from build123d import *

# Parameters (mm, degrees)
SKETCH1_W           = 10
SKETCH1_H           = 74.74
SKETCH1_R           = 2.05
BOSS_EXTRUDE1_DEPTH = 85
SKETCH1_2_R         = 2.05
BOSS_EXTRUDE2_DEPTH = 75
SKETCH2_R           = 1.75
CUT_EXTRUDE1_DEPTH  = 8
SKETCH3_R           = 1.75
CUT_EXTRUDE2_DEPTH  = 8


with BuildPart() as part:
    # Sketch1 → Boss-Extrude1 (new, symmetric)
    with BuildSketch(Plane(origin=(0, 0, 0), x_dir=(0, 0, -1), z_dir=(1, 0, 0))):
        Rectangle(SKETCH1_W, SKETCH1_H)
        with Locations((0, 30)):
            Circle(SKETCH1_R, mode=Mode.SUBTRACT)
        with Locations((0, -30)):
            Circle(SKETCH1_R, mode=Mode.SUBTRACT)
        Circle(SKETCH1_R, mode=Mode.SUBTRACT)
    extrude(amount=BOSS_EXTRUDE1_DEPTH, both=True)

    # Sketch1_2 → Boss-Extrude2 (add, symmetric)
    with BuildSketch(Plane(origin=(0, 0, 0), x_dir=(0, 0, -1), z_dir=(1, 0, 0))):
        with Locations((0, 30)):
            Circle(SKETCH1_2_R)
        Circle(SKETCH1_2_R)
        with Locations((0, -30)):
            Circle(SKETCH1_2_R)
    extrude(amount=BOSS_EXTRUDE2_DEPTH, both=True)

    # Sketch2 → Cut-Extrude1 (cut)
    with BuildSketch(Plane(origin=(0, 0, -5), x_dir=(-1, 0, 0), z_dir=(0, 0, -1))):
        with Locations(Location((-37, 22, 0), (0, 0, 90))):
            Circle(SKETCH2_R)
        with Locations(Location((37, 22, 0), (0, 0, 90))):
            Circle(SKETCH2_R)
        with Locations(Location((37, -22, 0), (0, 0, 90))):
            Circle(SKETCH2_R)
        with Locations(Location((-37, -22, 0), (0, 0, 90))):
            Circle(SKETCH2_R)
    extrude(amount=-CUT_EXTRUDE1_DEPTH, mode=Mode.SUBTRACT)

    # Sketch3 → Cut-Extrude2 (cut)
    with BuildSketch(Plane(origin=(0, 0, -5), x_dir=(-1, 0, 0), z_dir=(0, 0, -1))):
        with Locations(Location((-29, 24.5, 0), (0, 0, 90))):
            Circle(SKETCH3_R)
        with Locations(Location((29, 24.5, 0), (0, 0, 90))):
            Circle(SKETCH3_R)
        with Locations(Location((29, -24.5, 0), (0, 0, 90))):
            Circle(SKETCH3_R)
        with Locations(Location((-29, -24.5, 0), (0, 0, 90))):
            Circle(SKETCH3_R)
    extrude(amount=-CUT_EXTRUDE2_DEPTH, mode=Mode.SUBTRACT)


solid = part.part
Verification items for the finished model (mm, model axes). A direction names the side the tool comes from. Coordinates: 2 decimals unless noted, no trailing zeros. Loops run counter-clockwise (first coordinate to the right, second up) from the corner with the lowest first, then second, coordinate; pieces in that order, holes last. Notation, with made-up numbers: (62, 51) -> (108, 51) arc R27 cw to (108, 70) -> close; hole circle Ø1 at (84.25, 52.25). An arc over 180 degrees is marked (long way). Answer as a JSON object with one key per item and string values. Group by question number.
Item 1: Sectioned sample at B-B on y = 0. Record the boundary of the cut face in (x, z).
Item 2: Sectioned sample at C-C on z = 0.5. State how many separate pieces and enclosed holes the cut face has, plus the area to 3 significant figures.
Item 3: Depth check by flat-ended pin: pin 1 (1 mm diameter, centred on x = 36, y = 22, fed in from -Z); pin 2 (4 mm diameter, centred on x = -29, y = 25, fed in from -Z); pin 3 (3.5 mm diameter, centred on y = -30, z = 0, fed in from -X); pin 4 (2.5 mm diameter, centred on y = 30, z = 0, fed in from +X). Enter the tip coordinate at first touch or a pass-through.
Item 4: Scan lines: probe 1 along X at (y, z) = (-22, 0); probe 2 along X at (y, z) = (-24.5, -2); probe 3 along Y at (x, z) = (-38, -0.25). Record each from-to range of solid material in increasing order.
Item 5: Tool access check on faces 4 (the flat face through (37, -22, 3)), 5 (the flat face through (75, -30, 0)), 6 (the cylindrical face through (-80.07, 32.033, 0.267)). Record the directions out of +Z, -Z, +X, -X, +Y, -Y that give a thin tool (end or side, any length) a straight path to the whole face; none if there is none.
Item 6: Mould release check, pull along Y, two halves, no side actions. Record for faces 1 (the cylindrical face through (79.93, 32.033, 0.267)), 2 (the flat face through (1, -1, 5)), 3 (the flat face through (1, -37.37, 0)): +Y half, -Y half, draft (parallel to the pull), parting line (faces both ways), or undercut.
Item 7: Sectioned sample at A-A on x = -29. Record the boundary of the cut face in (y, z), plus the area to 3 significant figures.
Evaluation:
{
 "1": {"outline": "(-85, -5) -> (85, -5) -> (85, -2.05) -> (75, -2.05) -> (75, 2.05) -> (85, 2.05) -> (85, 5) -> (-85, 5) -> (-85, 2.05) -> (-75, 2.05) -> (-75, -2.05) -> (-85, -2.05) -> close"},
 "2": {"separate pieces": "1", "enclosed holes": "8", "area": "12,400 mm²"},
 "3": {"pin 1": "stops at z = 3", "pin 2": "stops at z = -5", "pin 3": "stops at x = -75", "pin 4": "stops at x = 75"},
 "4": {"probe 1": "x = -85 to -38.75, -35.25 to 35.25, 38.75 to 85", "probe 2": "x = -85 to -30.75, -27.25 to 27.25, 30.75 to 85", "probe 3": "y = -37.37 to -23.44, -20.56 to 20.56, 23.44 to 37.37"},
 "5": {"face 4": "-Z", "face 5": "+X", "face 6": "-X"},
 "6": {"face 1": "undercut", "face 2": "draft", "face 3": "-Y half"},
 "7": {"outline": "(-37.37, -5) -> (-26.25, -5) -> (-26.25, 3) -> (-22.75, 3) -> (-22.75, -5) -> (22.75, -5) -> (22.75, 3) -> (26.25, 3) -> (26.25, -5) -> (37.37, -5) -> (37.37, 5) -> (-37.37, 5) -> close", "area": "691 mm²"}
}
